Read the model definition and answer for the solid it produces. Units are mm, in the model's axes. A direction names the side the tool comes from. Give positions to 0.01 mm unless a question says otherwise; leave off trailing zeros. Write each loop counter-clockwise with the first axis right and the second up, starting at its lowest first coordinate (ties: lowest second). Pieces come first, ordered by that corner, then holes. Notation, with made-up numbers: (-31, -2) -> (2, -2) arc R29 cw to (2, 26) -> close; hole circle Ø7 at (64.25, 36). An arc over 180 degrees is marked (long way). Answer as CSV lines item,"result". Start each with the question number.
1. The part is cut by section A-A, the plane y = -6. Determine the outline of the cut face in (x, z), and give its area (3 significant figures).
2. A tool of negligible diameter and unlimited length cuts with its end or side. For faces 1 (the flat face through (-25.4, -3.8, 26.6)), 2 (the flat face through (26.4, -5, 0)), 3 (the flat face through (-25.4, -3.8, -26.6)), 4 (the flat face through (0, -5, -26.4)), from which of +Z, -Z, +X, -X, +Y, -Y can it reach the whole face along a straight path? Write none if from no direction.
3. Find the intervals of material crossed by line 1 (Z direction, x = -8, y = -2.5); line 2 (Y direction, x = 24, z = 12.5), in increasing order.
4. The part is cut by section C-C, the plane z = -12.5. Determine the outline of the cut face in (x, y), and give its area (3 significant figures).
5. Given pin 1 (1 mm diameter, centred on x = 20, z = -13, fed in from -Y); pin 2 (1.4 mm diameter, centred on y = -2, z = -26.5, fed in from -X); pin 3 (0.8 mm diameter, centred on x = -26.5, y = -4, fed in from +Z); pin 4 (2 mm diameter, centred on x = -7.5, z = -20, fed in from +Y), each flat-ended and moving along its own axis, determine where each tip first touches the part or whether it passes through.
6. The part is cut by section B-B, the plane x = 1. Determine the outline of the cut face in (y, z), and give its area (3 significant figures).
7. For a pull along X with two mould halves and no side action, classify faces 5 (the flat face through (-26.4, -5, 0)), 6 (the cylindrical face through (0.356, -0.485, 26.589)), 7 (the flat face through (27.1, -5, 0)) as pulls with the +X half, pulls with the -X half, needs draft (parallel to the pull), parting line crosses it, or undercut.
from build123d import *

# Parameters (mm, degrees)
SKETCH1_W          = 50.8
SKETCH1_H          = 50.8
BASE_FLANGE1_DEPTH = 0.7
EDGE_FLANGE1_DEPTH = 50.8
EDGE_FLANGE2_DEPTH = 50.8
EDGE_FLANGE3_DEPTH = 50.8
EDGE_FLANGE4_DEPTH = 50.8


# Sheet-metal steps are written as plain solids
with BuildPart() as part:
    # Sketch1 → Base-Flange1 (new body)
    with BuildSketch(Plane(origin=(0, 0, 0), x_dir=(1, 0, 0), z_dir=(0, 1, 0))):
        Rectangle(SKETCH1_W, SKETCH1_H)
    extrude(amount=-BASE_FLANGE1_DEPTH)

    # Edge-Flange1 section (across the edge) → Edge-Flange1 (add)
    with BuildSketch(Plane(origin=(26.4, -0.7, -25.4), x_dir=(-1, 0, 0), z_dir=(0, 0, 1))):
        with BuildLine():
            Line((-0.7, 1), (-0.7, 6.8))
            Line((-0.7, 6.8), (0, 6.8))
            Line((0, 6.8), (0, 1))
            ThreePointArc((0, 1), (0.292893219, 0.292893219), (1, 0))
            Line((1, 0), (1, -0.7))
            ThreePointArc((1, -0.7), (-0.202081528, -0.202081528), (-0.7, 1))
        make_face()
    extrude(amount=EDGE_FLANGE1_DEPTH)

    # Edge-Flange2 section (across the edge) → Edge-Flange2 (add)
    with BuildSketch(Plane(origin=(25.4, -0.7, 26.4), x_dir=(0, 0, -1), z_dir=(-1, 0, 0))):
        with BuildLine():
            Line((-0.7, 1), (-0.7, 6.8))
            Line((-0.7, 6.8), (0, 6.8))
            Line((0, 6.8), (0, 1))
            ThreePointArc((0, 1), (0.292893219, 0.292893219), (1, 0))
            Line((1, 0), (1, -0.7))
            ThreePointArc((1, -0.7), (-0.202081528, -0.202081528), (-0.7, 1))
        make_face()
    extrude(amount=EDGE_FLANGE2_DEPTH)

    # Edge-Flange3 section (across the edge) → Edge-Flange3 (add)
    with BuildSketch(Plane(origin=(-26.4, -0.7, 25.4), x_dir=(1, 0, 0), z_dir=(0, 0, -1))):
        with BuildLine():
            Line((-0.7, 1), (-0.7, 6.8))
            Line((-0.7, 6.8), (0, 6.8))
            Line((0, 6.8), (0, 1))
            ThreePointArc((0, 1), (0.292893219, 0.292893219), (1, 0))
            Line((1, 0), (1, -0.7))
            ThreePointArc((1, -0.7), (-0.202081528, -0.202081528), (-0.7, 1))
        make_face()
    extrude(amount=EDGE_FLANGE3_DEPTH)

    # Edge-Flange4 section (across the edge) → Edge-Flange4 (add)
    with BuildSketch(Plane(origin=(-25.4, -0.7, -26.4), x_dir=(0, 0, 1), z_dir=(1, 0, 0))):
        with BuildLine():
            Line((-0.7, 1), (-0.7, 6.8))
            Line((-0.7, 6.8), (0, 6.8))
            Line((0, 6.8), (0, 1))
            ThreePointArc((0, 1), (0.292893219, 0.292893219), (1, 0))
            Line((1, 0), (1, -0.7))
            ThreePointArc((1, -0.7), (-0.202081528, -0.202081528), (-0.7, 1))
        make_face()
    extrude(amount=EDGE_FLANGE4_DEPTH)


solid = part.part
Results found:
1,outline,"(-27.1, -25.4) -> (-26.4, -25.4) -> (-26.4, 25.4) -> (-27.1, 25.4) -> close; (-25.4, -27.1) -> (25.4, -27.1) -> (25.4, -26.4) -> (-25.4, -26.4) -> close; (-25.4, 26.4) -> (25.4, 26.4) -> (25.4, 27.1) -> (-25.4, 27.1) -> close; (26.4, -25.4) -> (27.1, -25.4) -> (27.1, 25.4) -> (26.4, 25.4) -> close"
1,area,"142 mm²"
2,face 1,"+Z, -X, +Y, -Y"
2,face 2,"+Z, -Z, -Y"
2,face 3,"-Z, -X, +Y, -Y"
2,face 4,"+X, -X, -Y"
3,line 1,"z = -27.1 to -26.4, 26.4 to 27.1"
3,line 2,"y = -0.7 to 0"
4,outline,"(-27.1, -7.5) -> (-26.4, -7.5) -> (-26.4, -1.7) arc R1 cw to (-25.4, -0.7) -> (25.4, -0.7) arc R1 cw to (26.4, -1.7) -> (26.4, -7.5) -> (27.1, -7.5) -> (27.1, -1.7) arc R1.7 ccw to (25.4, 0) -> (-25.4, 0) arc R1.7 ccw to (-27.1, -1.7) -> close"
4,area,"46.6 mm²"
5,pin 1,"stops at y = -0.7"
5,pin 2,"stops at x = -25.4"
5,pin 3,"stops at z = 25.4"
5,pin 4,"stops at y = 0"
6,outline,"(-7.5, -27.1) -> (-1.7, -27.1) arc R1.7 ccw to (0, -25.4) -> (0, 25.4) arc R1.7 ccw to (-1.7, 27.1) -> (-7.5, 27.1) -> (-7.5, 26.4) -> (-1.7, 26.4) arc R1 cw to (-0.7, 25.4) -> (-0.7, -25.4) arc R1 cw to (-1.7, -26.4) -> (-7.5, -26.4) -> close"
6,area,"46.6 mm²"
7,face 5,"undercut"
7,face 6,"needs draft"
7,face 7,"pulls with the +X half"
